Geometry check sheet. Reference: drawing and pictorial views, mm from the part's lowest x, y, z. Give positions to 0.01 mm unless a question says otherwise; leave off trailing zeros. Loops run counter-clockwise (first coordinate to the right, second up) from the corner with the lowest first, then second, coordinate; pieces in that order, holes last. Notation, with made-up numbers: (9.25, 23) - (61.25, 23) arc R33 cw to (61.25, 60) - close; hole circle Ø4 at (29.5, 9). An arc over 180 degrees is marked (long way). Put each result on its own line as item: value. Start each with the question number.
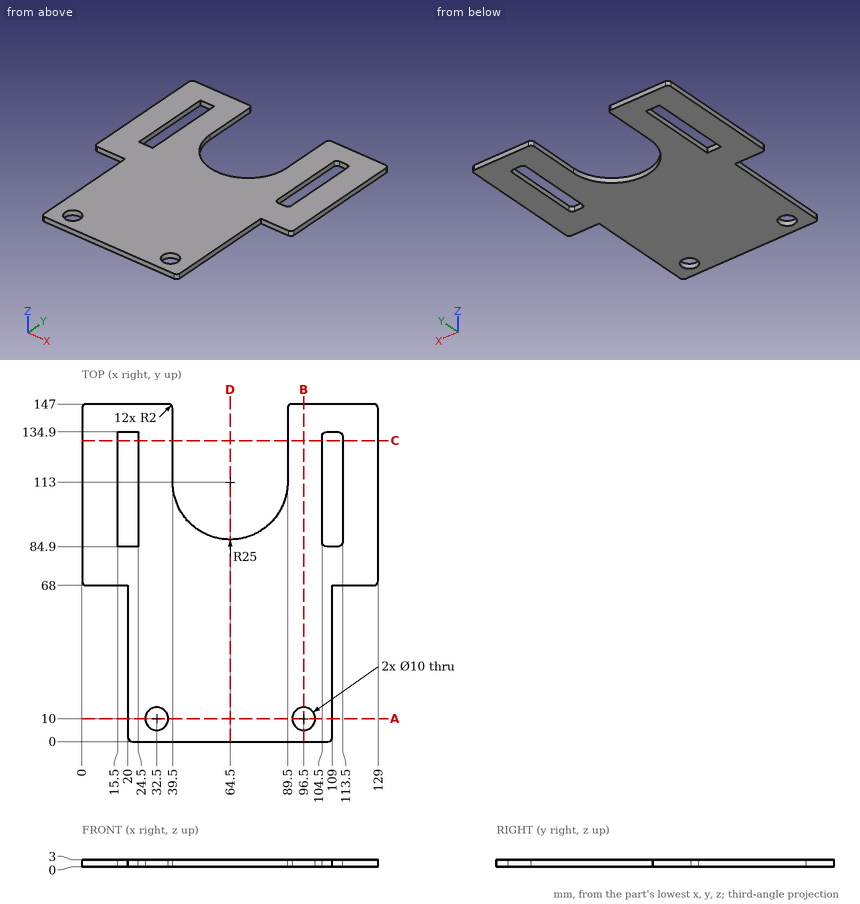
1) Depth check by flat-ended pin: P1, Ø1.5, axis at x = 116, z = 1, coming from the -Y side; P2, Ø0.9, axis at x = 109, z = 1, coming from the -Y side; P3, Ø0.9, axis at y = 47.5, z = 2, coming from the +X side. Enter the tip coordinate at first touch or a pass-through.
2) Section check C-C, the plane y = 131. Enter the section's corners in (x, z), plus the area to 3 significant figures.
3) Scan lines: line 1 along X through (y, z) = (126.5, 2.1); line 2 along Y through (x, z) = (32.5, 1.05); line 3 along X through (y, z) = (34, 0.1). Record each from-to range of solid material in increasing order. Write a range as from..to.
4) Section check A-A, the plane y = 10. Enter the section's corners in (x, z), plus the area to 3 significant figures.
5) Section check D-D, the plane x = 64.5. Enter the section's corners in (y, z).
6) Section check B-B, the plane x = 96.5. Enter the section's corners in (y, z).
Results are:
1. P1: stops at y = 68
1. P2: stops at y = 0.74
1. P3: stops at x = 109
2. outline: (0, 0) - (15.5, 0) - (15.5, 3) - (0, 3) - close; (24.5, 0) - (39.5, 0) - (39.5, 3) - (24.5, 3) - close; (89.5, 0) - (104.5, 0) - (104.5, 3) - (89.5, 3) - close; (113.5, 0) - (129, 0) - (129, 3) - (113.5, 3) - close
2. area: 183 mm2
3. line 1: x = 0..15.5, 24.5..39.5, 89.5..104.5, 113.5..129
3. line 2: y = 0..5, 15..147
3. line 3: x = 20..109
4. outline: (20, 0) - (27.5, 0) - (27.5, 3) - (20, 3) - close; (37.5, 0) - (91.5, 0) - (91.5, 3) - (37.5, 3) - close; (101.5, 0) - (109, 0) - (109, 3) - (101.5, 3) - close
4. area: 207 mm2
5. outline: (0, 0) - (88, 0) - (88, 3) - (0, 3) - close
6. outline: (0, 0) - (5, 0) - (5, 3) - (0, 3) - close; (15, 0) - (147, 0) - (147, 3) - (15, 3) - close
